```python
from build123d import *

# Parameters (mm, degrees)
SKETCH_1_R      = 8
SKETCH_1_R_2    = 1.5
SKETCH_1_W      = 20
SKETCH_1_H      = 3
SKETCH_1_W_2    = 6
EXTRUDE_1_DEPTH = 3


with BuildPart() as part:
    # 草图1 → 凸台-拉伸1 (new body)
    with BuildSketch(Plane(origin=(0, 0, 0), x_dir=(1, 0, 0), z_dir=(0, 1, 0))):
        with BuildLine():
            Line((-40, 0), (-40, 20))
            Line((-40, 20), (-40, 36))
            Line((-40, 36), (40, 36))
            Line((40, 36), (40, 20))
            Line((40, 20), (40, -15))
            ThreePointArc((40, -15), (38.535533906, -18.535533906), (35, -20))
            Line((35, -20), (0, -20))
            Line((0, -20), (-35, -20))
            ThreePointArc((-35, -20), (-38.535533906, -18.535533906), (-40, -15))
            Line((-40, -15), (-40, 0))
        make_face()
        with Locations(Location((16, 0, 0), (0, 0, 270))):
            Circle(SKETCH_1_R, mode=Mode.SUBTRACT)
        with Locations(Location((-16, 0, 0), (0, 0, 270))):
            Circle(SKETCH_1_R_2, mode=Mode.SUBTRACT)
        with Locations(Location((-35, 31, 0), (0, 0, 270))):
            Circle(SKETCH_1_R_2, mode=Mode.SUBTRACT)
        with Locations(Location((-35, 20, 0), (0, 0, 270))):
            Circle(SKETCH_1_R_2, mode=Mode.SUBTRACT)
        with Locations(Location((35, 20, 0), (0, 0, 270))):
            Circle(SKETCH_1_R_2, mode=Mode.SUBTRACT)
        with Locations(Location((35, 31, 0), (0, 0, 270))):
            Circle(SKETCH_1_R_2, mode=Mode.SUBTRACT)
        Polygon((-30, 20), (-10, 20), (-10, 23), (-20, 23), (-30, 23), align=None, mode=Mode.SUBTRACT)
        Polygon((10, 23), (10, 20), (30, 20), (30, 23), (20, 23), align=None, mode=Mode.SUBTRACT)
        with Locations((20, 29.5)):
            Rectangle(SKETCH_1_W, SKETCH_1_H, mode=Mode.SUBTRACT)
        with Locations((0, 29.5)):
            Rectangle(SKETCH_1_W_2, SKETCH_1_H, mode=Mode.SUBTRACT)
        with Locations((-20, 29.5)):
            Rectangle(SKETCH_1_W, SKETCH_1_H, mode=Mode.SUBTRACT)
        with Locations((0, 21.5)):
            Rectangle(SKETCH_1_W_2, SKETCH_1_H, mode=Mode.SUBTRACT)
    extrude(amount=EXTRUDE_1_DEPTH)


solid = part.part
```
Input: part model. Units: mm. Frame: model coordinates. A direction names the side the tool comes from. Coordinates: 2 decimals unless noted, no trailing zeros. Write each loop counter-clockwise with the first axis right and the second up, starting at its lowest first coordinate (ties: lowest second). Pieces come first, ordered by that corner, then holes.
1) Section D-D on y = 0.8. State how many separate pieces and enclosed holes the cut face has, and give its area (3 significant figures).
2) Set-up query: faces 1 (the flat face through (-1, 1, -36)), 2 (the flat face through (-20, 1, -20)). Return all of +Z, -Z, +X, -X, +Y, -Y with unobstructed straight access to the full face (end or side cutting, diameter ignored); none if empty.
3) Mould query, pull axis X, two halves, no side actions, for faces 3 (the flat face through (-3, 1, -29)), 4 (the flat face through (40, 1, -11)), 5 (the flat face through (1, 3, -8)), 6 (the flat face through (-40, 1, -10)). Classes: pulls with the +X half, pulls with the -X half, needs draft (parallel to the pull), parting line crosses it, or undercut.
4) Section A-A on x = 1. Output: boundary loops of the cut face in (y, z), and give its area (3 significant figures).
5) Section B-B on z = 0. Output: boundary loops of the cut face in (x, y), and give its area (3 significant figures).
6) Material intervals for line 1 along X through (y, z) = (1, 0); line 2 along Z through (x, y) = (-1, 2); line 3 along Z through (x, y) = (11, 2) (3 decimals), sorted ascending.
7) Pin query (flat end, axial travel): pin 1 Ø2.5 at (x, z) = (-35, -31) entering from +Y. Return the tip coordinate at first contact, or that it passes through.
8) Section C-C on x = 16. Output: boundary loops of the cut face in (y, z), and give its area (3 significant figures).
Check result:
1. separate pieces: 1
1. enclosed holes: 12
1. area: 3,960 mm2
2. face 1: -Z, +X, -X, +Y, -Y
2. face 2: +Y, -Y
3. face 3: undercut
3. face 4: pulls with the +X half
3. face 5: needs draft
3. face 6: pulls with the -X half
4. outline: (0, -36) - (3, -36) - (3, -31) - (0, -31) - close; (0, -28) - (3, -28) - (3, -23) - (0, -23) - close; (0, -20) - (3, -20) - (3, 20) - (0, 20) - close
4. area: 150 mm2
5. outline: (-40, 0) - (-17.5, 0) - (-17.5, 3) - (-40, 3) - close; (-14.5, 0) - (8, 0) - (8, 3) - (-14.5, 3) - close; (24, 0) - (40, 0) - (40, 3) - (24, 3) - close
5. area: 183 mm2
6. line 1: x = -40 to -17.5, -14.5 to 8, 24 to 40
6. line 2: z = -36 to -31, -28 to -23, -20 to 20
6. line 3: z = -36 to -31, -28 to -23, -20 to -6.245, 6.245 to 20
7. pin 1: passes through
8. outline: (0, -36) - (3, -36) - (3, -31) - (0, -31) - close; (0, -28) - (3, -28) - (3, -23) - (0, -23) - close; (0, -20) - (3, -20) - (3, -8) - (0, -8) - close; (0, 8) - (3, 8) - (3, 20) - (0, 20) - close
8. area: 102 mm2
